Geometry check sheet. Reference: the model listing, model coordinates, mm. A direction names the side the tool comes from. Coordinates: 2 decimals unless noted, no trailing zeros. Write each loop counter-clockwise with the first axis right and the second up, starting at its lowest first coordinate (ties: lowest second). Pieces come first, ordered by that corner, then holes. Notation, with made-up numbers: (69, -22.75) -> (74, -22.75) arc R23 ccw to (74, 16.25) -> close; hole circle Ø10 at (-36.75, 3.5). An arc over 180 degrees is marked (long way). Answer in a Markdown table with one row per item. Add a question column.
1. Depth check by flat-ended pin: P1, Ø6, axis at y = -8.5, z = 1.5, coming from the -X side; P2, Ø4, axis at x = 3, z = -1.5, coming from the -Y side; P3, Ø5, axis at y = 11.5, z = 1, coming from the -X side. Enter the tip coordinate at first touch or a pass-through.
2. Mould release check, pull along X, two halves, no side actions. Record for faces 3 (the cylindrical face through (11.952, 0.112, 5.03)), 4 (the flat face through (14.3, 3.4, 10.6)), 5 (the cylindrical face through (28.71, 4.48, 5.28)): pulls with the +X half, pulls with the -X half, needs draft (parallel to the pull), parting line crosses it, or undercut.
3. Cross-section at D-D on z = -2. Record the cut outline in (x, y).
4. Set-up check for faces 1 (the cylindrical face through (-0.85, 0.04, 0.46)), 2 (the flat face through (0, 0, -3)): record each of +Z, -Z, +X, -X, +Y, -Y from which the full face is reachable in a straight line by a thin tool's end or side.
5. Scan lines: L1, parallel to Y at x = 14.5, z = 2.5; L2, parallel to Z at x = 9, y = -3.5; L3, parallel to X at y = -1.25, z = 3.25. Record each from-to range of solid material in increasing order. Write a range as from..to.
6. Cross-section at A-A on y = 0. Record the cut outline in (x, z), and give its area (3 significant figures).
7. Cross-section at B-B on x = 14.5. Record the cut outline in (y, z).
8. Cross-section at C-C on z = 4.75. Record the cut outline in (x, y), and give its area (3 significant figures).
```python
from build123d import *

# Parameters (mm, degrees)
SKETCH_R          = 14.9
SKETCH_R_2        = 2.55
PAD_DEPTH         = 10.5
FILLET_R          = 0.5
SKETCH001_R       = 0.85
PAD001_DEPTH      = 5.25
PAD001_DEPTH_BACK = 3.5


with BuildPart() as fillet_body:
    # Sketch → Pad (new body)
    with BuildSketch(Plane.XY.offset(0.1)):
        with Locations((14.5, 0)):
            Circle(SKETCH_R)
        with Locations((14.5, 0)):
            Circle(SKETCH_R_2, mode=Mode.SUBTRACT)
    extrude(amount=PAD_DEPTH)

    # Fillet
    fillet_edges = [fillet_body.edges().sort_by_distance(p)[0] for p in [
        (11.95, 0, 10.6),
        (-0.4, 0, 10.6),
        (-0.4, 0, 0.1),
    ]]
    fillet(fillet_edges, radius=FILLET_R)


with BuildPart() as obj1:
    # Sketch001 → Pad001 (new body, two sides)
    with BuildSketch(Plane.XY.offset(0.5)) as pad001_sk:
        Circle(SKETCH001_R)
        with Locations((29, 0)):
            Circle(SKETCH001_R)
    extrude(amount=PAD001_DEPTH)
    extrude(pad001_sk.sketch, amount=-PAD001_DEPTH_BACK)

    # obj1: union Fillet body
    add(fillet_body.part)


solid = obj1.part
```
Results found:
| question | item | result |
|---|---|---|
| 1 | P1 | stops at x = 0.65 |
| 1 | P2 | stops at y = -10.34 |
| 1 | P3 | stops at x = 2.63 |
| 2 | face 3 | undercut |
| 2 | face 4 | needs draft |
| 2 | face 5 | parting line crosses it |
| 3 | outline | circle Ø1.7 at (0, 0); circle Ø1.7 at (29, 0) |
| 4 | face 1 | -Z |
| 4 | face 2 | -Z, +X, -X, +Y, -Y |
| 5 | L1 | y = -14.9..-2.55, 2.55..14.9 |
| 5 | L2 | z = 0.1..10.6 |
| 5 | L3 | x = -0.35..12.28, 16.72..29.35 |
| 6 | outline | (-0.85, -3) -> (0.85, -3) -> (0.85, 0.1) -> (11.95, 0.1) -> (11.95, 10.1) arc R0.5 ccw to (11.45, 10.6) -> (0.1, 10.6) arc R0.5 ccw to (-0.4, 10.1) -> (-0.4, 5.75) -> (-0.85, 5.75) -> close; (17.05, 0.1) -> (28.15, 0.1) -> (28.15, -3) -> (29.85, -3) -> (29.85, 5.75) -> (29.4, 5.75) -> (29.4, 10.1) arc R0.5 ccw to (28.9, 10.6) -> (17.55, 10.6) arc R0.5 ccw to (17.05, 10.1) -> close |
| 6 | area | 275 mm^2 |
| 7 | outline | (-14.9, 0.6) arc R0.5 ccw to (-14.4, 0.1) -> (-2.55, 0.1) -> (-2.55, 10.1) arc R0.5 ccw to (-3.05, 10.6) -> (-14.4, 10.6) arc R0.5 ccw to (-14.9, 10.1) -> close; (2.55, 0.1) -> (14.4, 0.1) arc R0.5 ccw to (14.9, 0.6) -> (14.9, 10.1) arc R0.5 ccw to (14.4, 10.6) -> (3.05, 10.6) arc R0.5 ccw to (2.55, 10.1) -> close |
| 8 | outline | (-0.38, -0.76) arc R14.9 ccw to (29.38, -0.76) arc R0.85 ccw to (29.38, 0.76) arc R14.9 ccw to (-0.38, 0.76) arc R0.85 ccw to start; hole circle Ø5.1 at (14.5, 0) |
| 8 | area | 678 mm^2 |
